Source: CAD feature listing. Evaluate the final solid. Frame: model axes, mm. Coordinates: 2 decimals unless noted, no trailing zeros. Write each loop counter-clockwise with the first axis right and the second up, starting at its lowest first coordinate (ties: lowest second). Pieces come first, ordered by that corner, then holes. Notation, with made-up numbers: (42.25, 58) -> (64.25, 58) arc R26 cw to (64.25, 80) -> close; hole circle Ø11 at (-38.75, 36.5). An arc over 180 degrees is marked (long way). One line per item, written item: value. Start each with the question number.
1. Line query: line 1 (Y direction, x = 170, z = 6.5). Output: solid intervals per line, ascending.
2. First-contact query: P1, Ø6.5, axis at x = 170, y = -95, coming from the +Z side. Flat tip, straight axial feed; report the tip coordinate or a pass-through.
3. Section query B-B, the plane y = 95. Output: boundary loops of the cut face in (x, z).
4. Section query A-A, the plane x = 170. Output: boundary loops of the cut face in (y, z), and give its area (3 significant figures).
5. Mould query, pull axis X, two halves, no side actions, for faces 1 (the flat face through (-200, -2, 5)), 2 (the cylindrical face through (165, 96.6, 4.9)), 3 (the flat face through (-3, -125, 5)). Classes: released by +X, released by -X, zero draft, split by the parting line, or undercut.
from build123d import *

# Parameters (mm, degrees)
SKIZZE1_W                          = 400
SKIZZE1_H                          = 250
AUFSATZ_LINEAR_AUSTRAGEN1_DEPTH    = 10
F_10_5_10_5_DURCHMESSER_BOHRUNG1_D = 10.5


with BuildPart() as part:
    # Skizze1 → Aufsatz-Linear austragen1 (new body)
    with BuildSketch(Plane.XY):
        Rectangle(SKIZZE1_W, SKIZZE1_H)
    extrude(amount=AUFSATZ_LINEAR_AUSTRAGEN1_DEPTH)

    # Ø10.5 (10.5) Durchmesser Bohrung1 (through all)
    with Locations(Plane.XY.offset(10)):
        with Locations((170, 95), (170, -95)):
            Hole(F_10_5_10_5_DURCHMESSER_BOHRUNG1_D / 2)


solid = part.part
Computed values:
1. line 1: y = -125 to -100.25, -89.75 to 89.75, 100.25 to 125
2. P1: passes through
3. outline: (-200, 0) -> (164.75, 0) -> (164.75, 10) -> (-200, 10) -> close; (175.25, 0) -> (200, 0) -> (200, 10) -> (175.25, 10) -> close
4. outline: (-125, 0) -> (-100.25, 0) -> (-100.25, 10) -> (-125, 10) -> close; (-89.75, 0) -> (89.75, 0) -> (89.75, 10) -> (-89.75, 10) -> close; (100.25, 0) -> (125, 0) -> (125, 10) -> (100.25, 10) -> close
4. area: 2,290 mm²
5. face 1: released by -X
5. face 2: undercut
5. face 3: zero draft
